Geometry check sheet. Reference: the model listing, model coordinates, mm. Face numbers are marked on the shaded views. Coordinates: 2 decimals unless noted, no trailing zeros. Write each loop counter-clockwise with the first axis right and the second up, starting at its lowest first coordinate (ties: lowest second). Pieces come first, ordered by that corner, then holes.
from build123d import *

# Parameters (mm, degrees)
SKETCH1_R           = 10
BOSS_EXTRUDE1_DEPTH = 15
SKETCH2_R           = 4
CUT_EXTRUDE1_DEPTH  = 34.166247904
FILLET1_R           = 1


with BuildPart() as part:
    # Sketch1 → Boss-Extrude1 (new, symmetric)
    with BuildSketch(Plane(origin=(0, 0, 0), x_dir=(1, 0, 0), z_dir=(0, 1, 0))):
        with Locations(Location((0, 0, 0), (0, 0, 270))):
            Circle(SKETCH1_R)
    extrude(amount=BOSS_EXTRUDE1_DEPTH, both=True)

    # Sketch2 → Cut-Extrude1 (cut, through all)
    with BuildSketch(Plane(origin=(0, 15, 0), x_dir=(1, 0, 0), z_dir=(0, 1, 0))):
        with Locations(Location((0, 0, 0), (0, 0, 270))):
            Circle(SKETCH2_R)
    extrude(amount=-CUT_EXTRUDE1_DEPTH, mode=Mode.SUBTRACT)

    # Fillet1
    fillet1_edges = [part.edges().sort_by_distance(p)[0] for p in [
        (0, -15, -10),
        (0, 15, -10),
    ]]
    fillet(fillet1_edges, radius=FILLET1_R)


solid = part.part
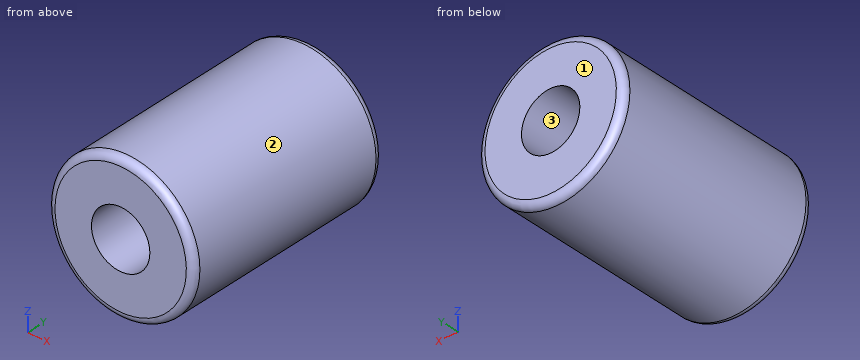
1. Gauge pin test, flat ends, axial feed: pin 1 Ø12 at (x, y) = (7, -0.5) entering from +Z; pin 2 Ø1.5 at (y, z) = (5.5, 4.5) entering from -X; pin 3 Ø8 at (x, y) = (8, 11) entering from -Z. Record the tip position at first contact, or that the pin passes through.
Computed values:
pin 1: stops at z = 9.95
pin 2: stops at x = -9.27
pin 3: stops at z = -9.17
2. Sectioned sample at A-A, the plane z = 0. Record the boundary of the cut face in (x, y).
Computed values:
outline: (-10, -14) arc R1 ccw to (-9, -15) - (-4, -15) - (-4, 15) - (-9, 15) arc R1 ccw to (-10, 14) - close; (4, -15) - (9, -15) arc R1 ccw to (10, -14) - (10, 14) arc R1 ccw to (9, 15) - (4, 15) - close
3. Draft check along Z on the marked faces 1, 2 and 3. Enter one of: released by +Z, released by -Z, zero draft, split by the parting line, or undercut.
Computed values:
face 1: zero draft
face 2: split by the parting line
face 3: undercut
4. Sectioned sample at C-C, the plane y = 8.75. Record the boundary of the cut face in (x, z), and give its area (3 significant figures).
Computed values:
outline: circle Ø20 at (0, 0); hole circle Ø8 at (0, 0)
area: 264 mm2
5. Thickness scan on line 1 along X through (y, z) = (4.75, 0); line 2 along X through (y, z) = (8, -1.75); line 3 along Z through (x, y) = (0.75, -2.5). Record the ranges inside material, lowest first.
Computed values:
line 1: x = -10 to -4, 4 to 10
line 2: x = -9.85 to -3.6, 3.6 to 9.85
line 3: z = -9.97 to -3.93, 3.93 to 9.97
6. Sectioned sample at B-B, the plane x = 0. Record the boundary of the cut face in (y, z), and give its area (3 significant figures).
Computed values:
outline: (-15, -9) arc R1 ccw to (-14, -10) - (14, -10) arc R1 ccw to (15, -9) - (15, -4) - (-15, -4) - close; (-15, 4) - (15, 4) - (15, 9) arc R1 ccw to (14, 10) - (-14, 10) arc R1 ccw to (-15, 9) - close
area: 359 mm2
